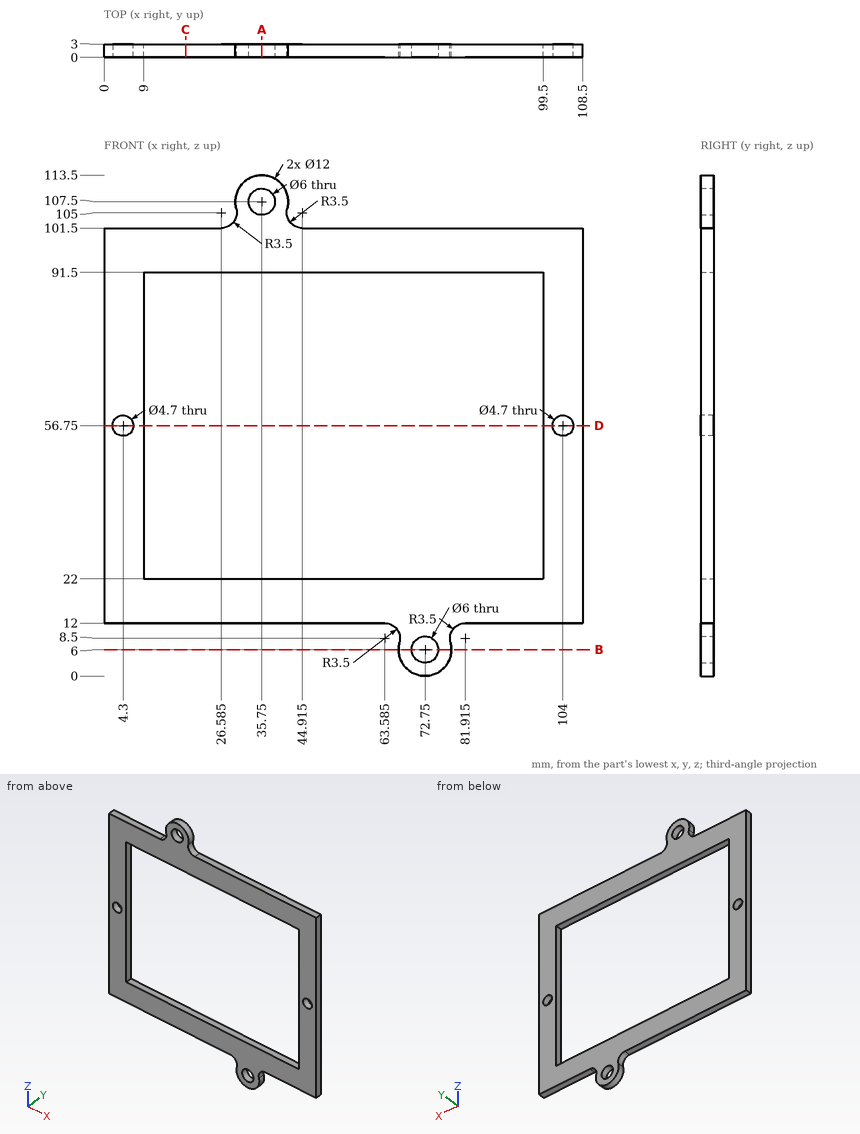
Study the drawing (mm; zero at the part's minimum x, y, z) and answer. Give positions to 0.01 mm unless a question says otherwise; leave off trailing zeros. Loops run counter-clockwise (first coordinate to the right, second up) from the corner with the lowest first, then second, coordinate; pieces in that order, holes last. Notation, with made-up numbers: M -21.75,-24.75 L 5.25,-24.75 A20 ccw 5.25,-2.75 Z; hole C -9,66.25 d7. An arc over 180 degrees is marked long. One line per item, written item: value.
1. Find the intervals of material crossed by probe 1 along Z at (x, y) = (35.75, 0.95); probe 2 along X at (y, z) = (1.85, 56.75); probe 3 along Z at (x, y) = (72.75, 1.35), in increasing order.
Found:
probe 1: 12 to 22, 91.5 to 104.5, 110.5 to 113.5
probe 2: 0 to 1.95, 6.65 to 9, 99.5 to 101.65, 106.35 to 108.5
probe 3: 0 to 3, 9 to 22, 91.5 to 101.5
2. Section D-D on z = 56.75 is taken. Determine the outline of the cut face in (x, y), plus the area to 3 significant figures.
Found:
outline: M 0,0 L 1.95,0 L 1.95,3 L 0,3 Z; M 6.65,0 L 9,0 L 9,3 L 6.65,3 Z; M 99.5,0 L 101.65,0 L 101.65,3 L 99.5,3 Z; M 106.35,0 L 108.5,0 L 108.5,3 L 106.35,3 Z
area: 25.8 mm^2
3. Section C-C on x = 18.5 is taken. Determine the outline of the cut face in (y, z), plus the area to 3 significant figures.
Found:
outline: M 0,12 L 3,12 L 3,22 L 0,22 Z; M 0,91.5 L 3,91.5 L 3,101.5 L 0,101.5 Z
area: 60.0 mm^2
4. Each of these flat-tipped pins is pushed along its axis until it touches: P1, Ø1.5, axis at x = 64, y = 1.5, coming from the -Z side; P2, Ø0.9, axis at x = 96, y = 1, coming from the -Z side; P3, Ø0.9, axis at x = 91.5, y = 2, coming from the +Z side. Where does it stop, or does it pass through?
Found:
P1: z = 11.8
P2: z = 12
P3: z = 101.5
5. Section A-A on x = 35.75 is taken. Determine the outline of the cut face in (y, z), plus the area to 3 significant figures.
Found:
outline: M 0,12 L 3,12 L 3,22 L 0,22 Z; M 0,91.5 L 3,91.5 L 3,104.5 L 0,104.5 Z; M 0,110.5 L 3,110.5 L 3,113.5 L 0,113.5 Z
area: 78.0 mm^2
6. Section B-B on z = 6 is taken. Determine the outline of the cut face in (x, y).
Found:
outline: M 66.75,0 L 69.75,0 L 69.75,3 L 66.75,3 Z; M 75.75,0 L 78.75,0 L 78.75,3 L 75.75,3 Z
